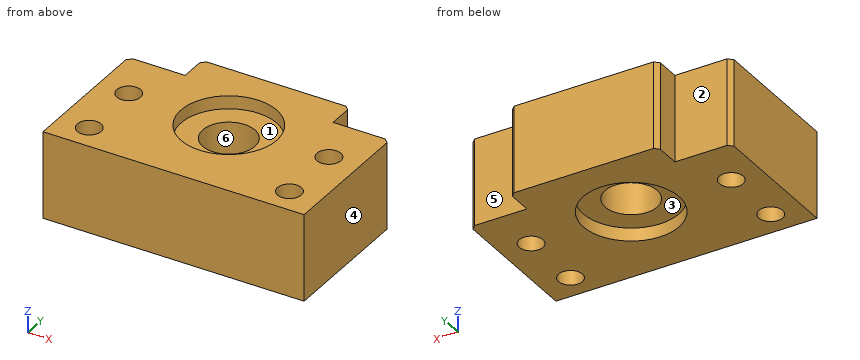
```python
from build123d import *

# Parameters (mm, degrees)
EXTRUDE_1_DEPTH     = 20
CHAMFER_1_SIZE      = 1
CHAMFER_2_SIZE      = 1
SKETCH_2_R          = 2.75
CUT_EXTRUDE_1_DEPTH = 20
SKETCH_4_R          = 6
CUT_EXTRUDE_2_DEPTH = 20
SKETCH_5_R          = 11
CUT_EXTRUDE_3_DEPTH = 3


with BuildPart() as part:
    # 草图1 → 凸台-拉伸1 (new body)
    with BuildSketch(Plane.XY):
        Polygon((-30, 0), (30, 0), (30, 32.5), (17, 32.5), (17, 39), (-17, 39), (-17, 32.5), (-30, 32.5), align=None)
    extrude(amount=EXTRUDE_1_DEPTH)

    # 倒角1
    chamfer_1_edges = [part.edges().sort_by_distance(p)[0] for p in [
        (17, 39, 10),
    ]]
    chamfer(chamfer_1_edges, length=CHAMFER_1_SIZE)

    # 倒角2
    chamfer_2_edges = [part.edges().sort_by_distance(p)[0] for p in [
        (-30, 32.5, 10),
        (-17, 39, 10),
        (30, 32.5, 10),
    ]]
    chamfer(chamfer_2_edges, length=CHAMFER_2_SIZE)

    # 草图2 → 切除-拉伸1 (cut)
    with BuildSketch(Plane.XY.offset(20)):
        with Locations((-23, 21)):
            Circle(SKETCH_2_R)
        with Locations((-23, 6)):
            Circle(SKETCH_2_R)
    cut_extrude_1 = extrude(amount=-CUT_EXTRUDE_1_DEPTH, mode=Mode.SUBTRACT)

    # 镜向1: 切除-拉伸1 across plane
    add(cut_extrude_1.mirror(Plane(origin=(0, 0, 0), x_dir=(0, 0, 1), z_dir=(1, 0, 0))), mode=Mode.SUBTRACT)

    # 草图4 → 切除-拉伸2 (cut)
    with BuildSketch(Plane.XY.offset(20)):
        with Locations((0, 21)):
            Circle(SKETCH_4_R)
    extrude(amount=-CUT_EXTRUDE_2_DEPTH, mode=Mode.SUBTRACT)

    # 草图5 → 切除-拉伸3 (cut)
    with BuildSketch(Plane.XY.offset(20)):
        with Locations((0, 21)):
            Circle(SKETCH_5_R)
    cut_extrude_3 = extrude(amount=-CUT_EXTRUDE_3_DEPTH, mode=Mode.SUBTRACT)

    # 镜向2: 切除-拉伸3 across plane
    add(cut_extrude_3.mirror(Plane(origin=(0, 0, 10), x_dir=(1, 0, 0), z_dir=(0, 0, -1))), mode=Mode.SUBTRACT)


solid = part.part
```
Model file for the job. Use its own axes, mm. Face numbers are marked on the shaded views. A direction names the side the tool comes from. Round coordinates to 2 decimals unless told otherwise and drop trailing zeros. Write each loop counter-clockwise with the first axis right and the second up, starting at its lowest first coordinate (ties: lowest second). Pieces come first, ordered by that corner, then holes. Notation, with made-up numbers: M 29,-19 L 60,-19 A23 cw 60,1 Z; hole C 9.5,46 d8. An arc over 180 degrees is marked long. Put each result on its own line as item: value.
Item 1: Cut at D-D (y = 6). List the corners of the cut face in (x, z), and give its area (3 significant figures).
Responses:
outline: M -30,0 L -25.75,0 L -25.75,20 L -30,20 Z; M -20.25,0 L 20.25,0 L 20.25,20 L -20.25,20 Z; M 25.75,0 L 30,0 L 30,20 L 25.75,20 Z
area: 980 mm²
Item 2: Flat gauge pins, fed straight in: P1, Ø11, axis at x = 3.5, y = 22, coming from the -Z side; P2, Ø5, axis at x = 10.5, z = 8.5, coming from the -Y side; P3, Ø11, axis at x = -0.5, y = 21.5, coming from the +Z side; P4, Ø6, axis at x = 21, z = 12, coming from the +Y side. Where does each tip first touch, or does it go through?
Responses:
P1: z = 3
P2: y = 0
P3: z = 17
P4: y = 32.5
Item 3: Cut at B-B (z = 18.25). List the corners of the cut face in (x, y).
Responses:
outline: M -30,0 L 30,0 L 30,31.5 L 29,32.5 L 17,32.5 L 17,38 L 16,39 L -16,39 L -17,38 L -17,32.5 L -29,32.5 L -30,31.5 Z; hole C -23,6 d5.5; hole C -23,21 d5.5; hole C 0,21 d22; hole C 23,6 d5.5; hole C 23,21 d5.5
Item 4: Cut at A-A (x = 23). List the corners of the cut face in (y, z).
Responses:
outline: M 0,0 L 3.25,0 L 3.25,20 L 0,20 Z; M 8.75,0 L 18.25,0 L 18.25,20 L 8.75,20 Z; M 23.75,0 L 32.5,0 L 32.5,20 L 23.75,20 Z
Item 5: Probe L1, parallel to Y at x = 23, z = 11; L2, parallel to Y at x = -22, z = 2.5; L3, parallel to Y at x = 0, z = 1.65. List the from-to ranges inside material, lowest first. Write a range as from..to.
Responses:
L1: 0..3.25, 8.75..18.25, 23.75..32.5
L2: 0..3.44, 8.56..18.44, 23.56..32.5
L3: 0..10, 32..39
Item 6: Mould opens along Y. For the marked faces 4, 5 and 6 say: +Y half, -Y half, draft (parallel to the pull), parting line (faces both ways), or undercut.
Responses:
face 4: draft
face 5: +Y half
face 6: undercut
Item 7: Tool access for the marked faces 1, 2 and 3: list every direction of +Z, -Z, +X, -X, +Y, -Y with a clear straight run to the whole face (end or side of a thin tool).
Responses:
face 1: +Z
face 2: +Z, -Z, -X, +Y
face 3: -Z
Item 8: Cut at C-C (y = 21). List the corners of the cut face in (x, z).
Responses:
outline: M -30,0 L -25.75,0 L -25.75,20 L -30,20 Z; M -20.25,0 L -11,0 L -11,3 L -6,3 L -6,17 L -11,17 L -11,20 L -20.25,20 Z; M 6,3 L 11,3 L 11,0 L 20.25,0 L 20.25,20 L 11,20 L 11,17 L 6,17 Z; M 25.75,0 L 30,0 L 30,20 L 25.75,20 Z
